```python
from build123d import *

# Parameters (mm, degrees)
BOSS_EXTRUDE1_DEPTH = 2.5
SKETCH2_R           = 1
CUT_EXTRUDE1_DEPTH  = 4.5
SKETCH3_R           = 1
CUT_EXTRUDE2_DEPTH  = 9.5
SKETCH5_R           = 1
BOSS_EXTRUDE2_DEPTH = 9.5
SKETCH7_W           = 2.5
SKETCH7_H           = 2.48697386
BOSS_EXTRUDE5_DEPTH = 17
SKETCH8_R           = 1
CUT_EXTRUDE3_DEPTH  = 9.5
SKETCH9_W           = 2.5
SKETCH9_H           = 2.510853282
CUT_EXTRUDE4_DEPTH  = 10.5
SKETCH10_R          = 1
CUT_EXTRUDE5_DEPTH  = 4.5
SKETCH11_R          = 1
BOSS_EXTRUDE6_DEPTH = 4.5
SKETCH12_R          = 1
CUT_EXTRUDE6_DEPTH  = 4
SKETCH13_W          = 2.5
SKETCH13_H          = 2.5
CUT_EXTRUDE7_DEPTH  = 6.5
SKETCH14_W          = 2.5
SKETCH14_H          = 2.5
BOSS_EXTRUDE7_DEPTH = 6.5
SKETCH15_R          = 1
CUT_EXTRUDE8_DEPTH  = 5
SKETCH16_R          = 1
BOSS_EXTRUDE8_DEPTH = 5
SKETCH17_W          = 2.5
SKETCH17_H          = 2.5
BOSS_EXTRUDE9_DEPTH = 17
SKETCH18_R          = 1
CUT_EXTRUDE9_DEPTH  = 5
SKETCH19_W          = 2.5
SKETCH19_H          = 2.5
CUT_EXTRUDE10_DEPTH = 6.3
SKETCH20_R          = 1
CUT_EXTRUDE11_DEPTH = 5


with BuildPart() as part:
    # Sketch1 → Boss-Extrude1 (new body)
    with BuildSketch(Plane.XY):
        Polygon((-70.406172668, -77.710060133), (-55.343173361, -77.710060133), (-55.155758053, -77.477979804), (-53.240646945, -79.084948828), (-54.148993857, -80.209773972), (-70.368347793, -80.209773972), align=None)
    extrude(amount=BOSS_EXTRUDE1_DEPTH)

    # Sketch2 → Cut-Extrude1 (cut)
    with BuildSketch(Plane(origin=(-60.939488189, -72.62485398, 0), x_dir=(0, 0, -1), z_dir=(0.6427876096865354, 0.7660444431189815, 0))):
        with Locations(Location((-1.25, -8.800123479, 0), (0, 0, 90))):
            Circle(SKETCH2_R)
    extrude(amount=-CUT_EXTRUDE1_DEPTH, mode=Mode.SUBTRACT)

    # Sketch3 → Cut-Extrude2 (cut)
    with BuildSketch(Plane(origin=(-71.565670343, -1.082908957, 0), x_dir=(0, 0, 1), z_dir=(-0.9998855357578962, -0.015129949839474955, 0))):
        with Locations(Location((1.25, -77.885923249, 0), (0, 0, 270))):
            Circle(SKETCH3_R)
    extrude(amount=-CUT_EXTRUDE2_DEPTH, mode=Mode.SUBTRACT)

    # Sketch5 → Boss-Extrude2 (add)
    with BuildSketch(Plane(origin=(-71.565670343, -1.082908957, 0), x_dir=(0, 0, 1), z_dir=(-0.9998855357578961, -0.015129949839476386, 0))):
        with Locations((1.25, -77.885923249)):
            Circle(SKETCH5_R)
    extrude(amount=-BOSS_EXTRUDE2_DEPTH)

    # Sketch7 → Boss-Extrude5 (add)
    with BuildSketch(Plane(origin=(-71.565670343, -1.082908957, 0), x_dir=(0, 0, 1), z_dir=(-0.9998855357578961, -0.015129949839476386, 0))):
        with Locations((1.25, -77.879410179)):
            Rectangle(SKETCH7_W, SKETCH7_H)
    extrude(amount=BOSS_EXTRUDE5_DEPTH)

    # Sketch8 → Cut-Extrude3 (cut)
    with BuildSketch(Plane(origin=(-88.56372445, -1.340118104, 0), x_dir=(0, 0, 1), z_dir=(-0.9998855357578962, -0.015129949839480206, 0))):
        with Locations(Location((1.25, -77.885923249, 0), (0, 0, 270))):
            Circle(SKETCH8_R)
    extrude(amount=-CUT_EXTRUDE3_DEPTH, mode=Mode.SUBTRACT)

    # Sketch9 → Cut-Extrude4 (cut)
    with BuildSketch(Plane(origin=(-88.56372445, -1.340118104, 0), x_dir=(0, 0, 1), z_dir=(-0.9998855357578962, -0.015129949839480206, 0))):
        with Locations((1.25, -77.89134989)):
            Rectangle(SKETCH9_W, SKETCH9_H)
    extrude(amount=-CUT_EXTRUDE4_DEPTH, mode=Mode.SUBTRACT)

    # Sketch10 → Cut-Extrude5 (cut)
    with BuildSketch(Plane(origin=(-78.064926325, -1.181253631, 0), x_dir=(0, 0, 1), z_dir=(-0.9998855357578961, -0.015129949839478678, 0))):
        with Locations(Location((1.25, -77.885923249, 0), (0, 0, 270))):
            Circle(SKETCH10_R)
    extrude(amount=-CUT_EXTRUDE5_DEPTH, mode=Mode.SUBTRACT)

    # Sketch11 → Boss-Extrude6 (add)
    with BuildSketch(Plane(origin=(-78.064926325, -1.181253631, 0), x_dir=(0, 0, 1), z_dir=(-0.9998855357578961, -0.015129949839478678, 0))):
        with Locations((1.25, -77.885923249)):
            Circle(SKETCH11_R)
    extrude(amount=-BOSS_EXTRUDE6_DEPTH)

    # Sketch12 → Cut-Extrude6 (cut)
    with BuildSketch(Plane(origin=(-78.064926325, -1.181253631, 0), x_dir=(0, 0, 1), z_dir=(-0.9998855357578961, -0.015129949839478678, 0))):
        with Locations(Location((1.25, -77.885923249, 0), (0, 0, 270))):
            Circle(SKETCH12_R)
    extrude(amount=-CUT_EXTRUDE6_DEPTH, mode=Mode.SUBTRACT)

    # Sketch13 → Cut-Extrude7 (cut)
    with BuildSketch(Plane(origin=(-78.064926325, -1.181253631, 0), x_dir=(0, 0, 1), z_dir=(-0.9998855357578961, -0.015129949839478678, 0))):
        with Locations((1.25, -77.885923249)):
            Rectangle(SKETCH13_W, SKETCH13_H)
    extrude(amount=-CUT_EXTRUDE7_DEPTH, mode=Mode.SUBTRACT)

    # Sketch14 → Boss-Extrude7 (add)
    with BuildSketch(Plane(origin=(-71.565670343, -1.082908957, 0), x_dir=(0, 0, 1), z_dir=(-0.9998855357578961, -0.015129949839476386, 0))):
        with Locations((1.25, -77.885923249)):
            Rectangle(SKETCH14_W, SKETCH14_H)
    extrude(amount=BOSS_EXTRUDE7_DEPTH)

    # Sketch15 → Cut-Extrude8 (cut)
    with BuildSketch(Plane(origin=(-78.064926325, -1.181253631, 0), x_dir=(0, 0, 1), z_dir=(-0.9998855357578961, -0.01512994983947622, 0))):
        with Locations(Location((1.25, -77.885923249, 0), (0, 0, 270))):
            Circle(SKETCH15_R)
    extrude(amount=-CUT_EXTRUDE8_DEPTH, mode=Mode.SUBTRACT)

    # Sketch16 → Boss-Extrude8 (add)
    with BuildSketch(Plane(origin=(-78.064926325, -1.181253631, 0), x_dir=(0, 0, 1), z_dir=(-0.9998855357578961, -0.01512994983947622, 0))):
        with Locations((1.25, -77.885923249)):
            Circle(SKETCH16_R)
    extrude(amount=-BOSS_EXTRUDE8_DEPTH)

    # Sketch17 → Boss-Extrude9 (add)
    with BuildSketch(Plane(origin=(-78.064926325, -1.181253631, 0), x_dir=(0, 0, 1), z_dir=(-0.9998855357578961, -0.01512994983947622, 0))):
        with Locations((1.25, -77.885923249)):
            Rectangle(SKETCH17_W, SKETCH17_H)
    extrude(amount=BOSS_EXTRUDE9_DEPTH)

    # Sketch18 → Cut-Extrude9 (cut)
    with BuildSketch(Plane(origin=(-95.062980433, -1.438462778, 0), x_dir=(0, 0, 1), z_dir=(-0.9998855357578961, -0.01512994983947622, 0))):
        with Locations(Location((1.25, -77.885923249, 0), (0, 0, 270))):
            Circle(SKETCH18_R)
    extrude(amount=-CUT_EXTRUDE9_DEPTH, mode=Mode.SUBTRACT)

    # Sketch19 → Cut-Extrude10 (cut)
    with BuildSketch(Plane(origin=(-95.062980433, -1.438462778, 0), x_dir=(0, 0, 1), z_dir=(-0.9998855357578961, -0.01512994983947622, 0))):
        with Locations((1.25, -77.885923249)):
            Rectangle(SKETCH19_W, SKETCH19_H)
    extrude(amount=-CUT_EXTRUDE10_DEPTH, mode=Mode.SUBTRACT)

    # Sketch20 → Cut-Extrude11 (cut)
    with BuildSketch(Plane(origin=(-88.763701558, -1.343144094, 0), x_dir=(0, 0, 1), z_dir=(-0.9998855357578961, -0.015129949839476473, 0))):
        with Locations(Location((1.25, -77.885923249, 0), (0, 0, 270))):
            Circle(SKETCH20_R)
    extrude(amount=-CUT_EXTRUDE11_DEPTH, mode=Mode.SUBTRACT)


solid = part.part
```
For this review, take the finished solid that the model builds, in its own axes (mm). A direction names the side the tool comes from. Give positions to 0.01 mm unless a question says otherwise; leave off trailing zeros. Order: outer loops, then holes, each group sorted by start corner. A loop starts at its lowest first (then second) coordinate and runs counter-clockwise, first axis right, second up.
1) Insertion check: pin 1 (1.2 mm diameter, centred on x = -64.5, z = 1.5, fed in from -Y). The pin has a flat end and moves straight along its axis. Give the tip position at first contact, or say it passes through.
2) Take a section at C-C (z = 0.7). Give the boundary of the cut face in (x, y), then the cut area to 3 significant figures.
3) Take a section at B-B (x = -62). Give the boundary of the cut face in (y, z).
4) Wall thickness on line 1 (Y direction, x = -63.5, z = 1.7); line 2 (Y direction, x = -83.5, z = 1.7); line 3 (X direction, y = -80.15, z = 0.65): over which ranges is each line inside the solid? List them lowest first.
5) Take a section at D-D (x = -80). Give the boundary of the cut face in (y, z), then the cut area to 3 significant figures.
6) The part is to be moulded in two halves that separate along X. For faces 5 (the face through (-53.69, -79.64, 1.23)), 6 (the face through (-55.75, -78.65, 1.55)), 7 (the face through (-70, -79, 0)), say which applies: released by +X, released by -X, zero draft, split by the parting line, or undercut.
7) For faces 1 (the face through (-85.107, -80.106, 0.867)), 2 (the face through (-70, -79, 2.5)), 3 (the face through (-63, -77.71, 1)), 4 (the face through (-62, -80.21, 1)), list the 3-axis set-ups (+Z, -Z, +X, -X, +Y, -Y) from which the entire face can be reached by the end or side of a thin tool; tool diameter is ignored.
8) Take a section at A-A (z = 1.95). Give the boundary of the cut face in (x, y).
Derived:
1. pin 1: stops at y = -80.21
2. outline: (-87.6, -78.39) - (-82.6, -78.31) - (-82.57, -79.98) - (-87.57, -80.06) - (-87.57, -80.47) - (-70.37, -80.21) - (-56.91, -80.21) - (-54.84, -77.74) - (-55.16, -77.48) - (-55.34, -77.71) - (-70.41, -77.71) - (-87.6, -77.97) - close; (-54.73, -80.21) - (-54.15, -80.21) - (-53.24, -79.08) - (-53.56, -78.82) - close
2. area: 71.7 mm2
3. outline: (-80.21, 0) - (-77.71, 0) - (-77.71, 2.5) - (-80.21, 2.5) - close
4. line 1: y = -80.21 to -77.71
4. line 2: y = -80.41 to -80.05, -78.27 to -77.91
4. line 3: x = -87.57 to -56.81, -54.72 to -54.1
5. outline: (-80.36, 0) - (-77.86, 0) - (-77.86, 2.5) - (-80.36, 2.5) - close
5. area: 6.25 mm2
6. face 5: released by +X
6. face 6: undercut
6. face 7: zero draft
7. face 1: none
7. face 2: +Z, +X, -X, +Y, -Y
7. face 3: +Z, -Z, -X, +Y
7. face 4: +Z, -Z, +X, -Y
8. outline: (-87.6, -78.51) - (-82.6, -78.43) - (-82.58, -79.86) - (-87.57, -79.93) - (-87.57, -80.47) - (-70.37, -80.21) - (-56.75, -80.21) - (-54.75, -77.82) - (-55.16, -77.48) - (-55.34, -77.71) - (-70.41, -77.71) - (-87.6, -77.97) - close; (-54.88, -80.21) - (-54.15, -80.21) - (-53.24, -79.08) - (-53.65, -78.74) - close
